The model under review builds one solid part; all positions refer to its coordinate system, in mm. Face numbers are marked on the shaded views. A direction names the side the tool comes from. Round coordinates to 2 decimals unless told otherwise and drop trailing zeros. Write each loop counter-clockwise with the first axis right and the second up, starting at its lowest first coordinate (ties: lowest second). Pieces come first, ordered by that corner, then holes.
Item 1: Add section B-B (x = 0.8). Give the boundary of the cut face in (y, z).
Item 2: Clearance check with flat-ended pins moving along their axes: pin 1 Ø0.8 at (x, z) = (0.5, -9.5) entering from +Y; pin 2 Ø0.6 at (x, y) = (3, 6) entering from +Z; pin 3 Ø0.8 at (y, z) = (4.5, -9) entering from +X. State where each tip first meets the part, or that it passes through.
Item 3: Machinability: for the marked faces 1, 2, 3, 4 and 5, which of the approach directions +Z, -Z, +X, -X, +Y, -Y give a long, thin tool a straight path to every point of the face, cutting with its end or side? Answer none if there is none.
Item 4: Add section C-C (z = -1.75). Give the boundary of the cut face in (x, y), plus the area to 3 significant figures.
Item 5: To check wall thickness, follow L1, parallel to Z at x = 2.6, y = 1.75; L2, parallel to Z at x = 3.35, y = 6.25; L3, parallel to X at y = 3.5, z = -6.5. State the ranges of each line that lie inside material, in increasing order.
Item 6: Add section D-D (x = 3.4). Give the boundary of the cut face in (y, z).
Item 7: Draft analysis for pull direction Z (two halves, no side actions). For the marked faces 6, 7 and 8, state which applies: +Z half, -Z half, draft (parallel to the pull), parting line (faces both ways), or undercut.
Item 8: Add section A-A (y = 5.25). Give the boundary of the cut face in (x, z).
```python
from build123d import *

# Parameters (mm, degrees)
SALIENTE_EXTRUIR1_DEPTH = 10
CORTAR_EXTRUIR1_DEPTH   = 1.5
CORTAR_EXTRUIR2_DEPTH   = 2
CORTAR_EXTRUIR3_REACH   = 8
CROQUIS5_W              = 7
CROQUIS5_H              = 2
CORTAR_EXTRUIR4_DEPTH   = 1.5
CORTAR_EXTRUIR5_DEPTH   = 2


with BuildPart() as part:
    # Croquis1 → Saliente-Extruir1 (new body)
    with BuildSketch(Plane.XY):
        Polygon((0, 0), (6, 0), (6, 3), (4, 3), (4, 7), (0, 7), align=None)
    extrude(amount=-SALIENTE_EXTRUIR1_DEPTH)

    # Croquis2 → Cortar-Extruir1 (cut)
    with BuildSketch(Plane.XY):
        Polygon((4, 3), (0, 6), (0, 7), (4, 7), align=None)
    extrude(amount=-CORTAR_EXTRUIR1_DEPTH, mode=Mode.SUBTRACT)

    # Croquis4 → Cortar-Extruir2 (cut)
    with BuildSketch(Plane(origin=(6, 0, 0), x_dir=(0, 0, -1), z_dir=(1, 0, 0))):
        Polygon((1.5, 3), (0, 0), (0, 3), align=None)
    extrude(amount=-CORTAR_EXTRUIR2_DEPTH, mode=Mode.SUBTRACT)

    # Croquis5 → Cortar-Extruir3 (cut, up to next)
    with BuildSketch(Plane(origin=(6, 0, 0), x_dir=(0, 0, -1), z_dir=(1, 0, 0)), mode=Mode.PRIVATE) as cortar_extruir3_sk1:
        with Locations((5, 1)):
            Rectangle(CROQUIS5_W, CROQUIS5_H)
    cortar_extruir3_tool1 = extrude(cortar_extruir3_sk1.sketch, amount=-CORTAR_EXTRUIR3_REACH, mode=Mode.PRIVATE) & part.part
    add(cortar_extruir3_tool1.solids().sort_by_distance((6, 1, -5))[0], mode=Mode.SUBTRACT)

    # Croquis6 → Cortar-Extruir4 (cut)
    with BuildSketch(Plane(origin=(0, 0, -10), x_dir=(-1, 0, 0), z_dir=(0, 0, -1))):
        Polygon((-4, 7), (0, 7), (0, 6), (-1, 6), (-1, 3), (-4, 3), align=None)
    extrude(amount=-CORTAR_EXTRUIR4_DEPTH, mode=Mode.SUBTRACT)

    # Croquis7 → Cortar-Extruir5 (cut, symmetric)
    with BuildSketch(Plane.XY.offset(-5)):
        Polygon((4, 5), (4, 7), (0, 7), align=None)
    extrude(amount=CORTAR_EXTRUIR5_DEPTH, both=True, mode=Mode.SUBTRACT)


solid = part.part
```
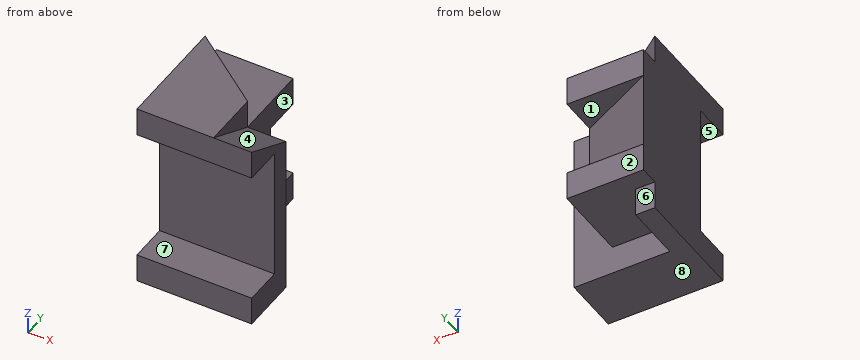
Numbers:
1. outline: (0, -10) - (6, -10) - (6, -8.5) - (7, -8.5) - (7, -7) - (6.6, -7) - (6.6, -3) - (7, -3) - (7, -1.5) - (5.4, -1.5) - (5.4, 0) - (0, 0) - (0, -1.5) - (2, -1.5) - (2, -8.5) - (0, -8.5) - close
2. pin 1: stops at y = 6
2. pin 2: stops at z = -1.5
2. pin 3: stops at x = 1
3. face 1: +X, +Y
3. face 2: +Z, -Z, +X, -X, +Y
3. face 3: +Z, -Z, +X, +Y
3. face 4: +Z, +X, +Y
3. face 5: +X, -X, -Y
4. outline: (0, 2) - (6, 2) - (6, 3) - (4, 3) - (4, 7) - (0, 7) - close
4. area: 22.0 mm2
5. L1: z = -10 to -8.5, -1.5 to 0
5. L2: z = -8.5 to -7, -3 to -1.5
5. L3: x = 0 to 4
6. outline: (0, -10) - (3, -10) - (3, -8.5) - (7, -8.5) - (7, -7) - (5.3, -7) - (5.3, -3) - (7, -3) - (7, -1.5) - (3.45, -1.5) - (3.45, 0) - (0, 0) - (0, -1.5) - (2, -1.5) - (2, -8.5) - (0, -8.5) - close
7. face 6: draft
7. face 7: undercut
7. face 8: -Z half
8. outline: (0, -10) - (1, -10) - (1, -8.5) - (4, -8.5) - (4, -7) - (3.5, -7) - (3.5, -3) - (4, -3) - (4, -1.5) - (1, -1.5) - (1, 0) - (0, 0) - close
